from build123d import *

# Parameters (mm, degrees)
BOSS_EXTRUDE1_DEPTH = 127
SKETCH2_R           = 30
CUT_EXTRUDE1_DEPTH  = 311.046770665
CHAMFER2_START      = -127
CHAMFER2_DEPTH      = 127


with BuildPart() as part:
    # Sketch1 → Boss-Extrude1 (new body)
    with BuildSketch(Plane(origin=(0, 0, 0), x_dir=(1, 0, 0), z_dir=(0, 1, 0))):
        with BuildLine():
            Line((48, 0), (200, 0))
            ThreePointArc((200, 0), (140.492634639, 142.344018533), (-2.618196121, 199.982861888))
            Line((-2.618196121, 199.982861888), (-2.618196121, 47.92854107))
            ThreePointArc((-2.618196121, 47.92854107), (33.002474045, 34.854507698), (48, 0))
        make_face()
    extrude(amount=-BOSS_EXTRUDE1_DEPTH)

    # Sketch2 → Cut-Extrude1 (cut, through all)
    with BuildSketch(Plane(origin=(0, 0, 0), x_dir=(1, 0, 0), z_dir=(0, 1, 0))):
        with Locations(Location((86.738855642, 88.590303092, 0), (0, 0, 270))):
            Circle(SKETCH2_R)
    extrude(amount=-CUT_EXTRUDE1_DEPTH, mode=Mode.SUBTRACT)

    # Chamfer2: read off the stored shape, not the designer's step
    # Chamfer2 outline → Chamfer2 (cut)
    with BuildSketch(Plane(origin=(0, 0, 0), x_dir=(1, 0, 0), z_dir=(0, 1, 0)).offset(CHAMFER2_START)):
        with BuildLine():
            ThreePointArc((200, 0), (199.983560067, 2.56431335), (199.93424297, 5.128205128))
            Line((199.93424297, 5.128205128), (194.935886896, 0))
            Line((194.935886896, 0), (200, 0))
        make_face()
        with BuildLine():
            Line((-2.618196121, 194.982861888), (2.384724212, 199.98578222))
            ThreePointArc((2.384724212, 199.98578222), (-0.116745086, 199.999965926), (-2.618196121, 199.982861888))
            Line((-2.618196121, 199.982861888), (-2.618196121, 194.982861888))
        make_face()
        with BuildLine():
            Line((48, 0), (52.763623833, 0))
            Line((52.763623833, 0), (47.785923471, 4.528301887))
            ThreePointArc((47.785923471, 4.528301887), (47.946450998, 2.266679661), (48, 0))
        make_face()
        with BuildLine():
            Line((2.682579438, 47.924980621), (-2.618196121, 52.676622021))
            Line((-2.618196121, 52.676622021), (-2.618196121, 47.92854107))
            ThreePointArc((-2.618196121, 47.92854107), (0.032240845, 47.999989172), (2.682579438, 47.924980621))
        make_face()
    extrude(amount=CHAMFER2_DEPTH, mode=Mode.SUBTRACT)

    # Chamfer2 2 outline → Chamfer2 2 (revolve, cut)
    with BuildSketch(Plane.XY):
        Polygon((200, -122), (195, -127), (200, -127), align=None)
        Polygon((48, -127), (53, -127), (48, -122), align=None)
        Polygon((195, 0), (200, -5), (200, 0), align=None)
        Polygon((48, 0), (48, -5), (53, 0), align=None)
    revolve(axis=Axis((0, 0, 0), (0, 1, 0)), mode=Mode.SUBTRACT)


solid = part.part
Here's how the part is built. I have some questions about the finished solid (model axes, mm). Coordinates: 2 decimals unless noted, no trailing zeros. Order: outer loops, then holes, each group sorted by start corner. A loop starts at its lowest first (then second) coordinate and runs counter-clockwise, first axis right, second up. Notation, with made-up numbers: (33.25, 74.5) -> (61.25, 74.5) arc R16 cw to (61.25, 80.5) -> close; hole circle Ø7 at (13.5, 88). An arc over 180 degrees is marked (long way). Answer in a Markdown table with one row per item.
(1) Will these pins go through, and if not, where does the flat tip stop? pin 1 Ø2 at (x, y) = (142.5, -84) entering from -Z; pin 2 Ø10 at (x, y) = (43, -69) entering from -Z; pin 3 Ø3 at (x, y) = (60.5, -49) entering from -Z; pin 4 Ø3 at (x, y) = (134, -34) entering from +Z.
Answer key:
| item | result |
|---|---|
| pin 1 | z = -141.34 |
| pin 2 | z = -196.36 |
| pin 3 | z = -191.1 |
| pin 4 | z = 0 |
(2) Thinking about a two-plate mould opening in X: for faces 1 (the face through (-0.2, -64.4, -197.4)), 2 (the face through (197.47, -64.39, -2.6)), 3 (the face through (116.484, -62.611, -92.496)), which applies, +X half, -X half, draft (parallel to the pull), parting line (faces both ways), or undercut?
Answer key:
| item | result |
|---|---|
| face 1 | -X half |
| face 2 | +X half |
| face 3 | undercut |
(3) Please list where these lines run through material, in increasing order: probe 1 along X at (y, z) = (-50, -109.5); probe 2 along X at (y, z) = (-5.5, -116); probe 3 along X at (y, z) = (-78, -148).
Answer key:
| item | result |
|---|---|
| probe 1 | -2.62 to 65.23, 108.25 to 167.36 |
| probe 2 | -2.62 to 74.54, 98.93 to 162.92 |
| probe 3 | -2.62 to 134.52 |
(4) I want a section at A-A on y = -19.5. List the corners of the cut face in (x, z) for me.
Answer key:
| item | result |
|---|---|
| outline | (-2.62, -194.98) -> (2.38, -199.99) arc R200 ccw to (199.93, -5.13) -> (194.94, 0) -> (52.76, 0) -> (47.79, -4.53) arc R48 cw to (2.68, -47.92) -> (-2.62, -52.68) -> close; hole circle Ø60 at (86.74, -88.59) |
